Source: three-view drawing plus pictorial views. Frame: mm from the lowest corner of the part. Coordinates: 2 decimals unless noted, no trailing zeros. Order: outer loops, then holes, each group sorted by start corner. A loop starts at its lowest first (then second) coordinate and runs counter-clockwise, first axis right, second up. Notation, with made-up numbers: (15, 43.5) -> (66, 43.5) arc R20 ccw to (66, 47.5) -> close; hole circle Ø1 at (34.5, 87.5). An arc over 180 degrees is marked (long way). Use one line per item in the form item = value. Start each with the question number.
1) Section query A-A on x = 23. Output: boundary loops of the cut face in (y, z) (3 decimals), then the cut area to 3 significant figures.
2) Ray query, line 1 along Y through (x, z) = (23, 0.8) (3 decimals); line 2 along Y through (x, z) = (22.5, 3.4); line 3 along Y through (x, z) = (14.5, 2.6). Return the intervals inside material, ascending.
3) Pin query (flat end, axial travel): pin 1 (2 mm diameter, centred on x = 18.5, y = 32, fed in from -Z); pin 2 (2.5 mm diameter, centred on x = 23, y = 13, fed in from -Z). Return the tip coordinate at first contact, or that it passes through.
4) Section query B-B on z = 1.2. Output: boundary loops of the cut face in (x, y) (3 decimals).
5) Section query D-D on y = 37. Output: boundary loops of the cut face in (x, z).
6) Section query C-C on y = 13. Output: boundary loops of the cut face in (x, z) (3 decimals), then the cut area to 3 significant figures.
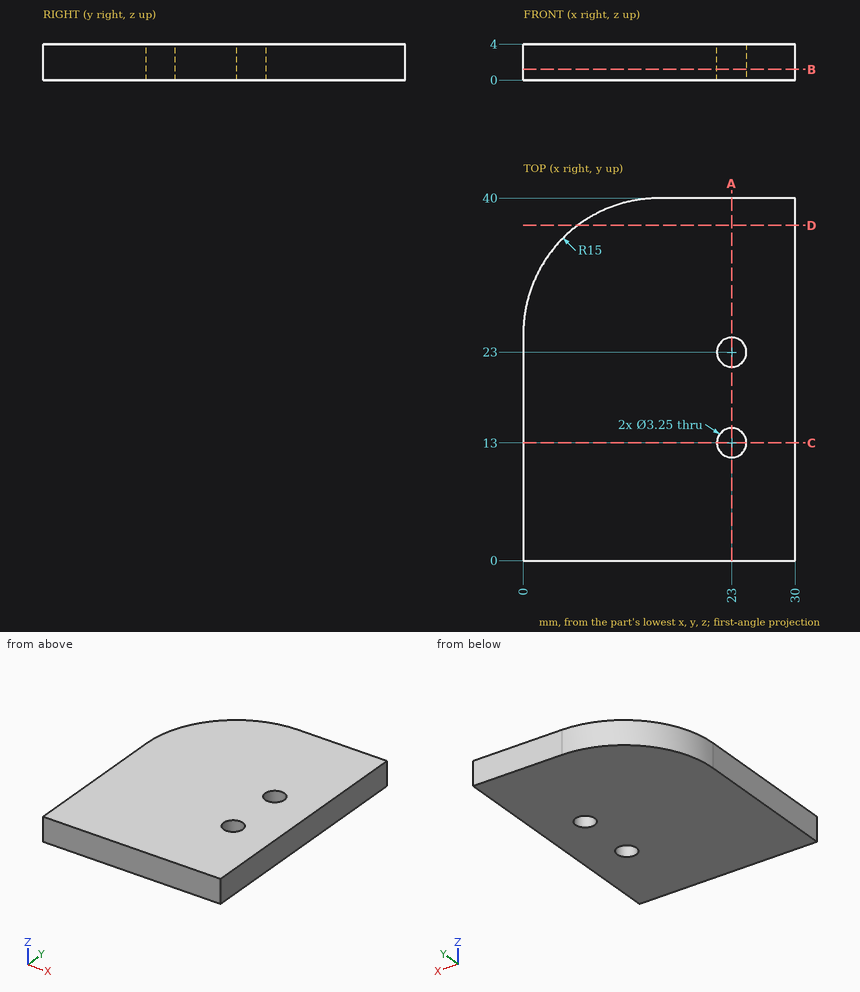
Answers below:
q1.outline = (0, 0) -> (11.375, 0) -> (11.375, 4) -> (0, 4) -> close; (14.625, 0) -> (21.375, 0) -> (21.375, 4) -> (14.625, 4) -> close; (24.625, 0) -> (40, 0) -> (40, 4) -> (24.625, 4) -> close
q1.area = 134 mm^2
q2.line_1 = 0 to 11.375, 14.625 to 21.375, 24.625 to 40
q2.line_2 = 0 to 11.45, 14.55 to 21.45, 24.55 to 40
q2.line_3 = 0 to 39.99
q3.pin_1 = 0
q3.pin_2 = through
q4.outline = (0, 0) -> (30, 0) -> (30, 40) -> (15, 40) arc R15 ccw to (0, 25) -> close; hole circle Ø3.25 at (23, 13); hole circle Ø3.25 at (23, 23)
q5.outline = (6, 0) -> (30, 0) -> (30, 4) -> (6, 4) -> close
q6.outline = (0, 0) -> (21.375, 0) -> (21.375, 4) -> (0, 4) -> close; (24.625, 0) -> (30, 0) -> (30, 4) -> (24.625, 4) -> close
q6.area = 107 mm^2
